Check sheet for the modelled part. Datum: model origin and axes. Units: mm. A direction names the side the tool comes from. Coordinates: 2 decimals unless noted, no trailing zeros. Order: outer loops, then holes, each group sorted by start corner. A loop starts at its lowest first (then second) coordinate and runs counter-clockwise, first axis right, second up.
from build123d import *

# Parameters (mm, degrees)
BOSS_EXTRUDE1_DEPTH             = 10
CUT_EXTRUDE1_DEPTH              = 28.408940147
CUT_EXTRUDE2_DEPTH              = 28.408940147
SKETCH4_W                       = 4
SKETCH4_H                       = 10
SKETCH5_W                       = 2
SKETCH5_H                       = 20.25
F_4_0_4_DIAMETER_HOLE2_D        = 4
F_4_0_4_DIAMETER_HOLE2_DEPTH    = 20.25
M7X1_0_TAPPED_HOLE1_D           = 6
M7X1_0_TAPPED_HOLE1_CBORE_D     = 7
M7X1_0_TAPPED_HOLE1_CBORE_DEPTH = 5
FILLET1_R                       = 5
CHAMFER1_SIZE                   = 1
CHAMFER1_SIZE2                  = 0.487732589
CHAMFER2_SIZE                   = 0.4
CHAMFER3_SIZE                   = 1
CHAMFER3_SIZE2                  = 0.487732589


with BuildPart() as part:
    # Sketch1 → Boss-Extrude1 (new body)
    with BuildSketch(Plane.XY.offset(10)):
        with BuildLine():
            Line((-9, -7.5), (-9, -14.5))
            Line((-9, -14.5), (9, -14.5))
            Line((9, -14.5), (9, -7.5))
            Line((9, -7.5), (17.529062862, -4.760458672))
            ThreePointArc((17.529062862, -4.760458672), (21, 0), (17.529062862, 4.760458672))
            Line((17.529062862, 4.760458672), (2.773364341, 9.5))
            Line((2.773364341, 9.5), (-2.773364341, 9.5))
            Line((-2.773364341, 9.5), (-17.529062862, 4.760458672))
            ThreePointArc((-17.529062862, 4.760458672), (-21, 0), (-17.529062862, -4.760458672))
            Line((-17.529062862, -4.760458672), (-9, -7.5))
        make_face()
    extrude(amount=-BOSS_EXTRUDE1_DEPTH)

    # Sketch2 → Cut-Extrude1 (cut, through all)
    with BuildSketch(Plane(origin=(0, 0, 0), x_dir=(-1, 0, 0), z_dir=(0, 0, -1))):
        Polygon((9, -11.230940108), (9, -10.769059892), (8.6, -11), align=None)
    extrude(amount=-CUT_EXTRUDE1_DEPTH, mode=Mode.SUBTRACT)

    # Sketch3 → Cut-Extrude2 (cut, through all)
    with BuildSketch(Plane(origin=(0, 0, 0), x_dir=(-1, 0, 0), z_dir=(0, 0, -1))):
        with BuildLine():
            Line((0.75, -14.5), (0.75, -3.929058411))
            ThreePointArc((0.75, -3.929058411), (0, -4), (-0.75, -3.929058411))
            Line((-0.75, -3.929058411), (-0.75, -14.5))
            Line((-0.75, -14.5), (0.75, -14.5))
        make_face()
    extrude(amount=-CUT_EXTRUDE2_DEPTH, mode=Mode.SUBTRACT)

    # Sketch4 → Cut-Revolve1 (revolve, cut)
    with BuildSketch(Plane.XZ):
        with Locations((2, 5)):
            Rectangle(SKETCH4_W, SKETCH4_H)
    revolve(axis=Axis((0, 0, 10), (0, 0, -1)), mode=Mode.SUBTRACT)

    # Sketch5 → Ø4.0 (4) Diameter Hole1 (revolve, cut)
    with BuildSketch(Plane(origin=(-0.75, -11, 5), x_dir=(0, 0, -1), z_dir=(0, 1, 0))):
        with Locations((1, 10.125)):
            Rectangle(SKETCH5_W, SKETCH5_H)
    revolve(axis=Axis((5.6, -11, 5), (-1, 0, 0)), mode=Mode.SUBTRACT)

    # Ø4.0 (4) Diameter Hole2
    with Locations(Plane.ZY.offset(-0.75)):
        with Locations((5, -11)):
            Hole(F_4_0_4_DIAMETER_HOLE2_D / 2, depth=F_4_0_4_DIAMETER_HOLE2_DEPTH)

    # M7x1.0 Tapped Hole1 (through all)
    with Locations(Plane.XY.offset(10)):
        with Locations((-16, 0), (16, 0)):
            CounterBoreHole(M7X1_0_TAPPED_HOLE1_D / 2, M7X1_0_TAPPED_HOLE1_CBORE_D / 2, M7X1_0_TAPPED_HOLE1_CBORE_DEPTH)

    # Fillet1
    fillet1_edges = [part.edges().sort_by_distance(p)[0] for p in [
        (-2.773364341, 9.5, 5),
        (2.773364341, 9.5, 5),
    ]]
    fillet(fillet1_edges, radius=FILLET1_R)

    # Chamfer1
    chamfer1_edges = [part.edges().sort_by_distance(p)[0] for p in [
        (12.5, 0, 10),
        (-19.5, 0, 10),
    ]]
    chamfer1_side = [part.faces().sort_by_distance(p)[0] for p in [
        (0, 9.016264535, 10),
    ]]
    chamfer(chamfer1_edges, length=CHAMFER1_SIZE, length2=CHAMFER1_SIZE2, reference=chamfer1_side[0])

    # Chamfer2
    chamfer2_edges = [part.edges().sort_by_distance(p)[0] for p in [
        (13.264531431, -6.130229336, 0),
        (21, 0, 0),
        (10.524097746, 7.010458672, 0),
        (2.763925905, 9.439751682, 0),
        (0, 9.5, 0),
        (-2.763925905, 9.439751682, 0),
        (-10.524097746, 7.010458672, 0),
        (-13.264531431, -6.130229336, 0),
        (-21, 0, 0),
        (-9, -9.134529946, 10),
        (-13.264531431, -6.130229336, 10),
        (-21, 0, 10),
        (-10.524097746, 7.010458672, 10),
        (-2.763925905, 9.439751682, 10),
        (0, 9.5, 10),
        (2.763925905, 9.439751682, 10),
        (10.524097746, 7.010458672, 10),
        (21, 0, 10),
        (13.264531431, -6.130229336, 10),
        (9, -11, 10),
        (4.875, -14.5, 10),
        (9, -14.5, 5),
        (0.75, -14.5, 5),
        (4.875, -14.5, 0),
        (0, 4, 10),
        (-9, -12.865470054, 10),
        (-9, -14.5, 5),
        (-4.875, -14.5, 0),
        (-0.75, -14.5, 5),
        (-4.875, -14.5, 10),
        (0, 4, 0),
    ]]
    chamfer(chamfer2_edges, length=CHAMFER2_SIZE - 0.0001)  # a hair under: the kernel refuses the full size

    # Chamfer3
    chamfer3_edges = [part.edges().sort_by_distance(p)[0] for p in [
        (19, 0, 0),
        (-13, 0, 0),
    ]]
    chamfer3_side = [part.faces().sort_by_distance(p)[0] for p in [
        (4.875, -13.627267497, 0),
    ]]
    chamfer(chamfer3_edges, length=CHAMFER3_SIZE, length2=CHAMFER3_SIZE2, reference=chamfer3_side[0])


solid = part.part
(1) Cross-section at A-A (y = -12.5). Enter the section's corners in (x, z), and give its area (3 significant figures).
Filled in:
outline: (-9, 0) - (-0.75, 0) - (-0.75, 3.68) - (-9, 3.68) - close; (-9, 6.32) - (-0.75, 6.32) - (-0.75, 10) - (-8.6, 10) - (-9, 9.6) - close; (0.75, 0) - (9, 0) - (9, 3.68) - (0.75, 3.68) - close; (0.75, 6.32) - (9, 6.32) - (9, 9.6) - (8.6, 10) - (0.75, 10) - close
area: 121 mm2
(2) Release check for a two-part mould opening along Y. For faces 3 (the cylindrical face through (-21, 0, 5)), 4 (the cylindrical face through (2.75, 9.44, 4.94)), 5 (the flat face through (19, 1, 5)), 6 (the flat face through (13.14, -5.96, 0.2)) record: +Y half, -Y half, draft (parallel to the pull), parting line (faces both ways), or undercut.
Filled in:
face 3: parting line
face 4: +Y half
face 5: undercut
face 6: -Y half
(3) Tool access check on faces 1 (the flat face through (0.75, -8, 5)), 2 (the flat face through (-13.127, -5.967, 9.797)). Record the directions out of +Z, -Z, +X, -X, +Y, -Y that give a thin tool (end or side, any length) a straight path to the whole face; none if there is none.
Filled in:
face 1: +Z, -Z, -Y
face 2: +Z, -X, -Y
(4) Cross-section at D-D (x = 0). Enter the section's corners in (y, z).
Filled in:
outline: (4, 0.4) - (4.4, 0) - (9.1, 0) - (9.5, 0.4) - (9.5, 9.6) - (9.1, 10) - (4.4, 10) - (4, 9.6) - close
(5) Cross-section at C-C (z = 8). Enter the section's corners in (x, y), and give its area (3 significant figures).
Filled in:
outline: (-17.53, -4.76) - (-9, -7.5) - (-9, -10.77) - (-8.6, -11) - (-9, -11.23) - (-9, -14.1) - (-8.6, -14.5) - (-1.15, -14.5) - (-0.75, -14.1) - (-0.75, -3.93) arc R4 cw (long way) to (0.75, -3.93) - (0.75, -14.1) - (1.15, -14.5) - (8.6, -14.5) - (9, -14.1) - (9, -7.5) - (17.53, -4.76) arc R5 ccw to (17.53, 4.76) - (3.52, 9.26) arc R5 ccw to (1.99, 9.5) - (-1.99, 9.5) arc R5 ccw to (-3.52, 9.26) - (-17.53, 4.76) arc R5 ccw to start; hole circle Ø7 at (-16, 0); hole circle Ø7 at (16, 0)
area: 534 mm2
(6) Thickness scan on probe 1 along Y at (x, z) = (3.5, 5); probe 2 along X at (y, z) = (-3, 7); probe 3 along X at (y, z) = (-8.75, 8). Record the ranges inside material, lowest first.
Filled in:
probe 1: y = -14.5 to -13, -9 to -1.94, 1.94 to 9.27
probe 2: x = -20 to -17.8, -14.2 to -2.65, 2.65 to 14.2, 17.8 to 20
probe 3: x = -9 to -0.75, 0.75 to 9
(7) Cross-section at B-B (x = -7.5). Enter the section's corners in (y, z), and give its area (3 significant figures).
Filled in:
outline: (-14.5, 0.4) - (-14.1, 0) - (7.56, 0) - (7.98, 0.4) - (7.98, 9.6) - (7.56, 10) - (-14.1, 10) - (-14.5, 9.6) - close; hole circle Ø4 at (-11, 5)
area: 212 mm2
(8) Go/stop test with flat-tipped pins: P1, Ø5, axis at y = -11, z = 5, coming from the +X side; P2, Ø0.9, axis at y = -12.5, z = 2.5, coming from the -X side; P3, Ø2, axis at x = -12.5, z = 1, coming from the +Y side. Record where each tip stops, or that it passes through.
Filled in:
P1: stops at x = 9
P2: stops at x = -9
P3: stops at y = 6.7
